Geometry check sheet. Reference: the model listing, model coordinates, mm. A direction names the side the tool comes from. Round coordinates to 2 decimals unless told otherwise and drop trailing zeros. Write each loop counter-clockwise with the first axis right and the second up, starting at its lowest first coordinate (ties: lowest second). Pieces come first, ordered by that corner, then holes. Notation, with made-up numbers: M 55.25,38 L 100.25,38 A30 ccw 100.25,63 Z; hole C -30,-35.5 d11. An arc over 180 degrees is marked long. One line per item, written item: value. Start each with the question number.
1. Section check B-B (z = -7). Record the boundary of the cut face in (x, y).
2. Release check for a two-part mould opening along X. For faces 4 (the cylindrical face through (0.86, 1.52, -0.9)), 5 (the cylindrical face through (20.2, 1.479, -50.693)), 6 (the flat face through (12, 1, -60)) record: pulls with the +X half, pulls with the -X half, needs draft (parallel to the pull), parting line crosses it, or undercut.
3. Access from +Z, -Z, +X, -X, +Y, -Y to the whole of each face (thin tool, end or side, straight path). Record for faces 1 (the flat face through (-10, 2, -20)), 2 (the flat face through (35, 2, -40)), 3 (the flat face through (0, 1, -50)).
4. Scan lines: probe 1 along X at (y, z) = (0.75, -30); probe 2 along Z at (x, y) = (6, 0.7); probe 3 along X at (y, z) = (1.35, -7). Record each from-to range of solid material in increasing order. Write a range as [from, to].
5. Depth check by flat-ended pin: P1, Ø3, axis at x = 6, z = -7, coming from the -Y side; P2, Ø0.9, axis at y = 2, z = -13, coming from the +X side; P3, Ø0.9, axis at x = 36, y = 1.5, coming from the -Z side; P4, Ø1.5, axis at y = 1, z = -15.5, coming from the -X side. Enter the tip coordinate at first touch or a pass-through.
6. Section check D-D (y = 2.3). Count the separate pieces of the cut face and the enclosed holes in it, and give its area (3 significant figures).
7. Section check A-A (x = 7). Record the boundary of the cut face in (y, z), and give its area (3 significant figures).
8. Section check C-C (x = -15). Record the boundary of the cut face in (y, z), and give its area (3 significant figures).
from build123d import *

# Parameters (mm, degrees)
SKETCH_1_W      = 25
SKETCH_1_H      = 60
SKETCH_1_R      = 2.6
EXTRUDE_1_DEPTH = 3
SKETCH_2_W      = 20
SKETCH_2_H      = 20
SKETCH_2_R      = 1.6
SKETCH_2_W_2    = 19.75
EXTRUDE_2_DEPTH = 3
FILLET_1_R      = 3


with BuildPart() as part:
    # 草图1 → 凸台-拉伸1 (new body)
    with BuildSketch(Plane(origin=(0, 0, 0), x_dir=(1, 0, 0), z_dir=(0, 1, 0))):
        with Locations((12.5, 30)):
            Rectangle(SKETCH_1_W, SKETCH_1_H)
        with Locations((6, 7)):
            Circle(SKETCH_1_R, mode=Mode.SUBTRACT)
        with Locations((19, 7)):
            Circle(SKETCH_1_R, mode=Mode.SUBTRACT)
        with Locations((6, 53)):
            Circle(SKETCH_1_R, mode=Mode.SUBTRACT)
        with Locations((19, 53)):
            Circle(SKETCH_1_R, mode=Mode.SUBTRACT)
    extrude(amount=EXTRUDE_1_DEPTH)

    # 草图2 → 凸台-拉伸2 (add)
    with BuildSketch(Plane(origin=(0, 3, 0), x_dir=(1, 0, 0), z_dir=(0, 1, 0))):
        with Locations((-10, 30)):
            Rectangle(SKETCH_2_W, SKETCH_2_H)
        with Locations((-15, 30)):
            Circle(SKETCH_2_R, mode=Mode.SUBTRACT)
        with Locations((34.875, 30)):
            Rectangle(SKETCH_2_W_2, SKETCH_2_H)
        with Locations((39.75, 30)):
            Circle(SKETCH_2_R, mode=Mode.SUBTRACT)
    extrude(amount=-EXTRUDE_2_DEPTH)

    # 圆角1
    fillet_1_edges = [part.edges().sort_by_distance(p)[0] for p in [
        (0, 1.5, -40),
        (0, 1.5, -20),
        (-20, 1.5, -20),
        (-20, 1.5, -40),
        (25, 1.5, -20),
        (25, 1.5, -40),
        (44.75, 1.5, -40),
        (44.75, 1.5, -20),
        (0, 1.5, -60),
        (25, 1.5, -60),
        (25, 1.5, 0),
        (0, 1.5, 0),
    ]]
    fillet(fillet_1_edges, radius=FILLET_1_R)


solid = part.part
Result sheet:
1. outline: M 0,0 L 3.4,0 L 3.4,3 L 0,3 Z; M 8.6,0 L 16.4,0 L 16.4,3 L 8.6,3 Z; M 21.6,0 L 25,0 L 25,3 L 21.6,3 Z
2. face 4: pulls with the -X half
2. face 5: undercut
2. face 6: needs draft
3. face 1: +Z, -X, +Y, -Y
3. face 2: -Z, +X, +Y, -Y
3. face 3: -Z, -X, +Y, -Y
4. probe 1: x = [-20, -16.6], [-13.4, 38.15], [41.35, 44.75]
4. probe 2: z = [-60, -55.6], [-50.4, -9.6], [-4.4, 0]
4. probe 3: x = [0, 3.4], [8.6, 16.4], [21.6, 25]
5. P1: passes through
5. P2: stops at x = 25
5. P3: stops at z = -40
5. P4: stops at x = 0
6. separate pieces: 1
6. enclosed holes: 6
6. area: 2,190 mm2
7. outline: M 0,-60 L 3,-60 L 3,-55.4 L 0,-55.4 Z; M 0,-50.6 L 3,-50.6 L 3,-9.4 L 0,-9.4 Z; M 0,-4.6 L 3,-4.6 L 3,0 L 0,0 Z
7. area: 151 mm2
8. outline: M 0,-40 L 3,-40 L 3,-31.6 L 0,-31.6 Z; M 0,-28.4 L 3,-28.4 L 3,-20 L 0,-20 Z
8. area: 50.4 mm2
